Source: CAD feature listing. Evaluate the final solid. Frame: model axes, mm. A direction names the side the tool comes from. Round coordinates to 2 decimals unless told otherwise and drop trailing zeros. Loops run counter-clockwise (first coordinate to the right, second up) from the corner with the lowest first, then second, coordinate; pieces in that order, holes last. Notation, with made-up numbers: (3.5, 70.5) -> (19.5, 70.5) arc R11 cw to (19.5, 88.5) -> close; hole circle Ø8 at (-25.5, 57.5). An arc over 180 degrees is marked (long way). Write item = value, one per line.
from build123d import *

# Parameters (mm, degrees)
F0_W          = 10
F0_H          = 55
F0_R          = 2.5
F1_DEPTH      = 2
F2_W          = 30
F2_H          = 2
F2_W_2        = 10
F3_DEPTH      = 2
F4_DEPTH      = 12
F4_DEPTH_BACK = 18
F5_DEPTH      = 20
F6_R          = 2.5
F7_DEPTH      = 10


with BuildPart() as f1:
    # F0 (on Top) → F1 (new body)
    with BuildSketch(Plane.XY):
        Rectangle(F0_W, F0_H)
        with Locations((0, -20)):
            Circle(F0_R, mode=Mode.SUBTRACT)
        with Locations((0, -12)):
            Circle(F0_R, mode=Mode.SUBTRACT)
        with Locations((0, 12)):
            Circle(F0_R, mode=Mode.SUBTRACT)
        with Locations((0, 20)):
            Circle(F0_R, mode=Mode.SUBTRACT)
    extrude(amount=F1_DEPTH)

    # F2 (on face) → F3 (join)
    with BuildSketch(Plane(origin=(-5, 0, 0), x_dir=(0, -1, 0), z_dir=(-1, 0, 0))):
        with Locations((0, 1)):
            Rectangle(F2_W, F2_H)
        with Locations((-20, 1)):
            Rectangle(F2_W_2, F2_H)
        with Locations((20, 1)):
            Rectangle(F2_W_2, F2_H)
        with BuildLine():
            Line((-25, 25), (-25, 2))
            Line((-25, 2), (-15, 2))
            Line((-15, 2), (-15, 10.9861218113))
            ThreePointArc((-15, 10.9861218113), (-17.5, 20), (-15, 29.0138781887))
            Line((-15, 29.0138781887), (-15, 40))
            Line((-15, 40), (-25, 25))
        make_face()
        with BuildLine():
            Line((-15, 10.9861218113), (-15, 2))
            Line((-15, 2), (15, 2))
            Line((15, 2), (15, 10.9861218113))
            ThreePointArc((15, 10.9861218113), (0, 2.5), (-15, 10.9861218113))
        make_face()
        with BuildLine():
            Line((15, 10.9861218113), (15, 2))
            Line((15, 2), (25, 2))
            Line((25, 2), (25, 25))
            Line((25, 25), (15, 40))
            Line((15, 40), (15, 29.0138781887))
            ThreePointArc((15, 29.0138781887), (16.863421954, 24.6770717335), (17.5, 20))
            ThreePointArc((17.5, 20), (16.863421954, 15.3229282665), (15, 10.9861218113))
        make_face()
        with BuildLine():
            Line((0, 40), (-15, 40))
            Line((-15, 40), (-15, 29.0138781887))
            ThreePointArc((-15, 29.0138781887), (0, 37.5), (15, 29.0138781887))
            Line((15, 29.0138781887), (15, 40))
            Line((15, 40), (0, 40))
        make_face()
    extrude(amount=F3_DEPTH)

    # F2 (on face) → F4 (join, two sides)
    with BuildSketch(Plane(origin=(-5, 0, 0), x_dir=(0, -1, 0), z_dir=(-1, 0, 0))) as f4_sk:
        with BuildLine():
            Line((-15, 29.0138781887), (-15, 10.9861218113))
            ThreePointArc((-15, 10.9861218113), (0, 2.5), (15, 10.9861218113))
            Line((15, 10.9861218113), (15, 29.0138781887))
            ThreePointArc((15, 29.0138781887), (0, 37.5), (-15, 29.0138781887))
        make_face()
        with BuildLine():
            Line((15, 29.0138781887), (15, 10.9861218113))
            ThreePointArc((15, 10.9861218113), (16.863421954, 15.3229282665), (17.5, 20))
            ThreePointArc((17.5, 20), (16.863421954, 24.6770717335), (15, 29.0138781887))
        make_face()
        with BuildLine():
            ThreePointArc((-15, 29.0138781887), (-17.5, 20), (-15, 10.9861218113))
            Line((-15, 10.9861218113), (-15, 29.0138781887))
        make_face()
    extrude(amount=-F4_DEPTH)
    extrude(f4_sk.sketch, amount=F4_DEPTH_BACK)

    # F2 (on face) → F5 (join)
    with BuildSketch(Plane(origin=(-5, 0, 0), x_dir=(0, -1, 0), z_dir=(-1, 0, 0))):
        with BuildLine():
            Line((-15, 10.9861218113), (-15, 2))
            Line((-15, 2), (15, 2))
            Line((15, 2), (15, 10.9861218113))
            ThreePointArc((15, 10.9861218113), (0, 2.5), (-15, 10.9861218113))
        make_face()
        with Locations((0, 1)):
            Rectangle(F2_W, F2_H)
    extrude(amount=F5_DEPTH)

    # F6 (on face) → F7 (join)
    with BuildSketch(Plane(origin=(0, 0, 0), x_dir=(1, 0, 0), z_dir=(0, 0, -1))):
        with Locations((-18, -7)):
            Circle(F6_R)
        with Locations((-18, 7)):
            Circle(F6_R)
    extrude(amount=F7_DEPTH)


solid = f1.part
1. Section query C-C (z = -2). Return the cut outline in (x, y).
Evaluation:
outline = circle Ø5 at (-18, -7); circle Ø5 at (-18, 7)
2. Contact query for flat-ended pins moving along their axis: pin 1 Ø12 at (x, z) = (-9.5, 17.5) entering from -Y; pin 2 Ø0.6 at (y, z) = (26, 1.5) entering from -X; pin 3 Ø8 at (x, z) = (-13, 7.5) entering from +Y. Output: stop coordinate, or through.
Evaluation:
pin_1 = -25
pin_2 = -5
pin_3 = 15.3
3. Section query D-D (x = -18). Return the cut outline in (y, z), then the cut area to 3 significant figures.
Evaluation:
outline = (-15, 0) -> (-9.5, 0) -> (-9.5, -10) -> (-4.5, -10) -> (-4.5, 0) -> (4.5, 0) -> (4.5, -10) -> (9.5, -10) -> (9.5, 0) -> (15, 0) -> (15, 10.99) arc R17.5 ccw (long way) to (-15, 10.99) -> close
area = 1,210 mm²
4. Set-up query: faces 1 (the face through (-5, 26, 1)), 2 (the face through (-23.99, -0.25, 2.5)), 3 (the face through (0, 0, 2)), 4 (the face through (-5, -26, 1)). Return all of +Z, -Z, +X, -X, +Y, -Y with unobstructed straight access to the full face (end or side cutting, diameter ignored); none if empty.
Evaluation:
face_1 = +Z, -Z, -X, +Y
face_2 = +Z, -X
face_3 = +X, +Y, -Y
face_4 = +Z, -Z, -X, -Y
5. Section query A-A (y = 20). Return the cut outline in (x, z), then the cut area to 3 significant figures.
Evaluation:
outline = (-7, 0) -> (-2.5, 0) -> (-2.5, 2) -> (-5, 2) -> (-5, 32.5) -> (-7, 32.5) -> close; (2.5, 0) -> (5, 0) -> (5, 2) -> (2.5, 2) -> close
area = 75.0 mm²
6. Line query: probe 1 along Y at (x, z) = (0, 0.95); probe 2 along X at (y, z) = (12, 37); probe 3 along X at (y, z) = (-6, 3). Output: solid intervals per line, ascending. Write a range as from..to.
Evaluation:
probe_1 = -27.5..-22.5, -17.5..-14.5, -9.5..9.5, 14.5..17.5, 22.5..27.5
probe_2 = -7..-5
probe_3 = -25..-5
7. Mould query, pull axis X, two halves, no side actions, for faces 5 (the face through (-25, 0, 2)), 6 (the face through (-0.54, -14.44, 0.99)), 7 (the face through (-0.33, 22.48, 0.99)), 8 (the face through (0, 27.5, 1)). Classes: released by +X, released by -X, zero draft, split by the parting line, or undercut.
Evaluation:
face_5 = released by -X
face_6 = undercut
face_7 = undercut
face_8 = zero draft
8. Section query B-B (x = 0). Return the cut outline in (y, z), then the cut area to 3 significant figures.
Evaluation:
outline = (-27.5, 0) -> (-22.5, 0) -> (-22.5, 2) -> (-27.5, 2) -> close; (-17.5, 0) -> (-14.5, 0) -> (-14.5, 2) -> (-17.5, 2) -> close; circle Ø35 at (0, 20); (-9.5, 0) -> (9.5, 0) -> (9.5, 2) -> (-9.5, 2) -> close; (14.5, 0) -> (17.5, 0) -> (17.5, 2) -> (14.5, 2) -> close; (22.5, 0) -> (27.5, 0) -> (27.5, 2) -> (22.5, 2) -> close
area = 1,030 mm²
